Can you work these out from the model? Positions are in its coordinate system, mm. Face numbers are marked on the shaded views. A direction names the side the tool comes from. Round coordinates to 2 decimals unless told otherwise and drop trailing zeros. Loops run counter-clockwise (first coordinate to the right, second up) from the corner with the lowest first, then second, coordinate; pieces in that order, holes last.
(1) Will these pins go through, and if not, where does the flat tip stop? pin 1 Ø2 at (x, z) = (-219, 170) entering from +Y; pin 2 Ø1.5 at (y, z) = (55, 164.5) entering from -X; pin 3 Ø22.5 at (y, z) = (53, 84.5) entering from -X; pin 4 Ø2.5 at (y, z) = (70.2, 167.9) entering from +X.
(2) I want a section at A-A on z = 152.4. Write out the boundary of the cut face in (x, y), plus the area to 3 significant figures.
(3) I want a section at C-C on x = -202. Write out the boundary of the cut face in (y, z), plus the area to 3 significant figures.
(4) Which directions (+Z, -Z, +X, -X, +Y, -Y) give clear straight access to the entire face, cutting with the end or side of a thin tool? Please do the marked faces 1 and 2.
(5) Thinking about a two-plate mould opening in X: for the marked faces 3, 4 and 5, which applies, released by +X, released by -X, zero draft, split by the parting line, or undercut?
(6) If I drill on line 1 along X through (y, z) = (3, 257); line 2 along Y through (x, z) = (-42, 191.5), over which ranges is the centre line in solid material (lowest first)?
(7) I want a section at B-B on z = 222.5. Write out the boundary of the cut face in (x, y), plus the area to 3 significant figures.
from build123d import *

# Parameters (mm, degrees)
F1_DEPTH  = 304.8
F2_R      = 3.69316
F3_R      = 1.98374
F4_W      = 1.70942
F4_H      = 43.0059846
F5_DEPTH  = 25.4
F6_R      = 11.2530001
F6_R_2    = 1.5
F7_DEPTH  = 1.70942
F8_SIZE   = 12.7
F9_R      = 1.8288
F10_DEPTH = 304.8


with BuildPart() as f1:
    # F0 (on Top) → F1 (new body)
    with BuildSketch(Plane.XY):
        Polygon((0, 50.8), (0, 0), (-301.38116, 0), (-301.38116, 50.8), (-303.09058, 50.8), (-303.09058, -1.70942), (1.70942, -1.70942), (1.70942, 50.8), align=None)
    extrude(amount=F1_DEPTH)

    # F2
    f2_edges = [f1.edges().sort_by_distance(p)[0] for p in [
        (1.70942, -1.70942, 152.4),
        (-303.09058, -1.70942, 152.4),
    ]]
    fillet(f2_edges, radius=F2_R)

    # F3
    f3_edges = [f1.edges().sort_by_distance(p)[0] for p in [
        (0, 0, 152.4),
        (-301.38116, 0, 152.4),
    ]]
    fillet(f3_edges, radius=F3_R)

    # F4 (on face) → F5 (join)
    with BuildSketch(Plane(origin=(0, 50.8, 0), x_dir=(-1, 0, 0), z_dir=(0, 1, 0))):
        with Locations((-0.85471, 152.4)):
            Rectangle(F4_W, F4_H)
    extrude(amount=F5_DEPTH)

    # F6 (on face) → F7 (cut, through all)
    with BuildSketch(Plane.YZ.offset(1.70942)):
        with Locations((54.6970077, 152.4)):
            Circle(F6_R)
        with Locations((70.1970021, 136.9000056)):
            Circle(F6_R_2)
        with Locations((39.1970133, 136.9000056)):
            Circle(F6_R_2)
        with Locations((39.1970133, 167.8999944)):
            Circle(F6_R_2)
        with Locations((70.1970021, 167.8999944)):
            Circle(F6_R_2)
    extrude(amount=-F7_DEPTH, mode=Mode.SUBTRACT)

    # F8
    f8_edges = [f1.edges().sort_by_distance(p)[0] for p in [
        (0.85471, 50.8, 0),
        (-302.23587, 50.8, 0),
        (-302.23587, 50.8, 304.8),
        (0.85471, 50.8, 304.8),
    ]]
    chamfer(f8_edges, length=F8_SIZE)

    # F9 (on face) → F10 (cut, through all)
    with BuildSketch(Plane.YZ.offset(1.70942)):
        with Locations((41.6436699622, 295.6436699622)):
            Circle(F9_R)
        with Locations((41.6436699622, 270.2436699622)):
            Circle(F9_R)
        with Locations((28.9436699622, 270.2436699622)):
            Circle(F9_R)
        with Locations((28.9436699622, 295.6436699622)):
            Circle(F9_R)
        with Locations((41.6436699622, 34.5563300378)):
            Circle(F9_R)
        with Locations((41.6436699622, 9.1563300378)):
            Circle(F9_R)
        with Locations((28.9436699622, 9.1563300378)):
            Circle(F9_R)
        with Locations((28.9436699622, 34.5563300378)):
            Circle(F9_R)
    extrude(amount=-F10_DEPTH, mode=Mode.SUBTRACT)


solid = f1.part
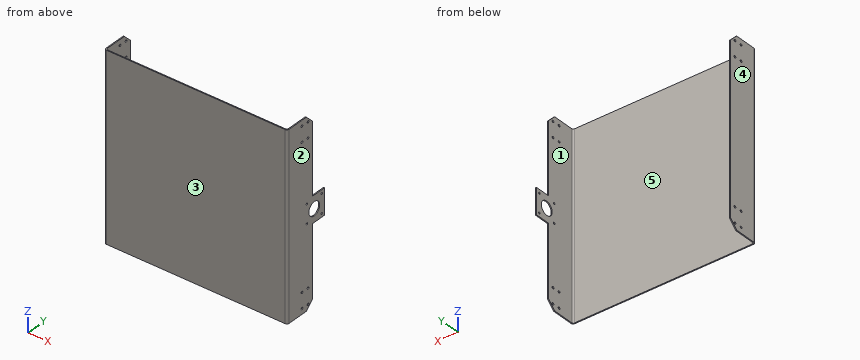
Filled sheet:
1. pin 1: stops at y = 0
1. pin 2: stops at x = 0
1. pin 3: stops at x = -303.09
1. pin 4: passes through
2. outline: (-303.09, 1.98) arc R3.69 ccw to (-299.4, -1.71) - (-1.98, -1.71) arc R3.69 ccw to (1.71, 1.98) - (1.71, 43.44) - (0, 43.44) - (0, 1.98) arc R1.98 cw to (-1.98, 0) - (-299.4, 0) arc R1.98 cw to (-301.38, 1.98) - (-301.38, 50.8) - (-303.09, 50.8) - close; (0, 65.95) - (1.71, 65.95) - (1.71, 76.2) - (0, 76.2) - close
2. area: 695 mm2
3. outline: (-1.71, 0) - (0, 0) - (0, 304.8) - (-1.71, 304.8) - close
3. area: 521 mm2
4. face 1: +Z, -Z, +Y
4. face 2: +Z, -Z, +X, +Y, -Y
5. face 3: zero draft
5. face 4: released by -X
5. face 5: undercut
6. line 1: x = -303.09 to -301.38, 0 to 1.71
6. line 2: y = -1.71 to 0
7. outline: (-303.09, 1.98) arc R3.69 ccw to (-299.4, -1.71) - (-1.98, -1.71) arc R3.69 ccw to (1.71, 1.98) - (1.71, 50.8) - (0, 50.8) - (0, 1.98) arc R1.98 cw to (-1.98, 0) - (-299.4, 0) arc R1.98 cw to (-301.38, 1.98) - (-301.38, 50.8) - (-303.09, 50.8) - close
7. area: 691 mm2
